from build123d import *

# Parameters (mm, degrees)
SKETCH1_W           = 120.65
SKETCH1_H           = 82.55
BOSS_EXTRUDE1_DEPTH = 12.7
FILLET1_R           = 16.002
SKETCH2_R           = 5.588
SKETCH2_R_2         = 3.231202494
SKETCH2_R_3         = 6.35
CUT_EXTRUDE1_DEPTH  = 12.7
BOSS_EXTRUDE2_START = 6.35
SKETCH2_5_W         = 25.4
SKETCH2_5_H         = 25.4
SKETCH2_5_R         = 6.35
BOSS_EXTRUDE2_DEPTH = 6.35
BOSS_EXTRUDE3_DEPTH = 25.4
BOSS_EXTRUDE4_DEPTH = 17.526
BOSS_EXTRUDE5_DEPTH = 12.7
FILLET2_R           = 3.175
FILLET3_R           = 3.175
FILLET4_R           = 3.175
SKETCH5_R           = 8.001
CUT_EXTRUDE2_DEPTH  = 4.572
SKETCH6_R           = 4.826
CUT_EXTRUDE3_DEPTH  = 25.654
SKETCH7_W           = 44.45
SKETCH7_H           = 12.7
CUT_EXTRUDE4_DEPTH  = 12.7
FILLET5_R           = 3.175
FILLET6_R           = 3.175
SKETCH8_R           = 3.175
CUT_EXTRUDE5_DEPTH  = 12.7


with BuildPart() as part:
    # Sketch1 → Boss-Extrude1 (new body)
    with BuildSketch(Plane(origin=(0, 0, 0), x_dir=(1, 0, 0), z_dir=(0, 1, 0))):
        Rectangle(SKETCH1_W, SKETCH1_H)
    extrude(amount=BOSS_EXTRUDE1_DEPTH)

    # Fillet1
    fillet1_edges = [part.edges().sort_by_distance(p)[0] for p in [
        (-60.325, 6.35, 41.275),
    ]]
    fillet(fillet1_edges, radius=FILLET1_R)

    # Sketch2 → Cut-Extrude1 (cut)
    with BuildSketch(Plane(origin=(0, 12.7, 0), x_dir=(1, 0, 0), z_dir=(0, 1, 0))):
        with Locations(Location((36.449, -9.525, 0), (0, 0, 270))):
            Circle(SKETCH2_R)
        with Locations(Location((36.449, -28.575, 0), (0, 0, 270))):
            Circle(SKETCH2_R)
        with Locations(Location((-9.525, 17.653, 0), (0, 0, 270))):
            Circle(SKETCH2_R_2)
        with Locations(Location((-44.323, -25.273, 0), (0, 0, 270))):
            Circle(SKETCH2_R)
        with Locations(Location((-3.175, -28.575, 0), (0, 0, 270))):
            Circle(SKETCH2_R_3)
        with BuildLine():
            Line((-47.625, 41.275), (-60.325, 41.275))
            Line((-60.325, 41.275), (-60.325, 28.575))
            ThreePointArc((-60.325, 28.575), (-51.344743879, 32.294743879), (-47.625, 41.275))
        make_face()
        with BuildLine():
            Line((-60.325, 3.175), (-31.877, 3.175))
            ThreePointArc((-31.877, 3.175), (-25.527, -3.175), (-31.877, -9.525))
            Line((-31.877, -9.525), (-60.325, -9.525))
            Line((-60.325, -9.525), (-60.325, 3.175))
        make_face()
    extrude(amount=-CUT_EXTRUDE1_DEPTH, mode=Mode.SUBTRACT)

    # Sketch2<5> → Boss-Extrude2 (add)
    with BuildSketch(Plane(origin=(0, 12.7, 0), x_dir=(1, 0, 0), z_dir=(0, 1, 0)).offset(BOSS_EXTRUDE2_START)):
        with Locations((-3.175, -28.575)):
            Rectangle(SKETCH2_5_W, SKETCH2_5_H)
        with Locations(Location((-3.175, -28.575, 0), (0, 0, 270))):
            Circle(SKETCH2_5_R, mode=Mode.SUBTRACT)
    extrude(amount=-BOSS_EXTRUDE2_DEPTH)

    # Sketch2<6> → Boss-Extrude3 (add)
    with BuildSketch(Plane(origin=(0, 12.7, 0), x_dir=(1, 0, 0), z_dir=(0, 1, 0))):
        Polygon((60.325, -41.275), (60.325, 41.275), (9.525, 41.275), (9.525, 28.575), (47.625, 28.575), (47.625, -41.275), align=None)
    extrude(amount=BOSS_EXTRUDE3_DEPTH)

    # Sketch2<10> → Boss-Extrude4 (add)
    with BuildSketch(Plane(origin=(0, 12.7, 0), x_dir=(1, 0, 0), z_dir=(0, 1, 0))):
        with BuildLine():
            Line((11.049, 28.575), (11.049, 14.351))
            ThreePointArc((11.049, 14.351), (23.749, 1.651), (36.449, 14.351))
            Line((36.449, 14.351), (36.449, 28.575))
            Line((36.449, 28.575), (11.049, 28.575))
        make_face()
    extrude(amount=BOSS_EXTRUDE4_DEPTH)

    # Sketch4 → Boss-Extrude5 (add)
    with BuildSketch(Plane(origin=(0, 0, -41.275), x_dir=(-1, 0, 0), z_dir=(0, 0, -1))):
        Polygon((-9.525, 38.1), (-9.525, 12.7), (34.469090512, 12.7), align=None)
    extrude(amount=-BOSS_EXTRUDE5_DEPTH)

    # Fillet2
    fillet2_edges = [part.edges().sort_by_distance(p)[0] for p in [
        (42.037, 12.7, -28.575),
        (36.449, 21.463, -28.575),
        (11.049, 12.7, -21.463),
        (11.049, 21.463, -28.575),
        (23.749, 12.7, -1.651),
        (36.449, 12.7, -21.463),
        (23.749, 30.226, -28.575),
        (-11.710045256, 12.7, -28.575),
        (47.625, 12.7, 6.35),
        (47.625, 25.4, -28.575),
    ]]
    fillet(fillet2_edges, radius=FILLET2_R)

    # Fillet3
    fillet3_edges = [part.edges().sort_by_distance(p)[0] for p in [
        (9.525, 15.875, 15.875),
        (-15.875, 15.875, 15.875),
        (-15.875, 15.875, 41.275),
        (9.525, 15.875, 41.275),
    ]]
    fillet(fillet3_edges, radius=FILLET3_R)

    # Fillet4
    # the kernel refuses this fillet: 3.175 mm, written as the material it adds along each edge
    with BuildSketch(Plane(origin=(9.525, 12.7, 19.05), x_dir=(0, 1, 0), z_dir=(0, 0, 1)), Plane(origin=(-12.7, 12.7, 15.875), x_dir=(0, 1, 0), z_dir=(1, 0, 0)), Plane(origin=(-15.875, 12.7, 38.1), x_dir=(0, 1, 0), z_dir=(0, 0, -1))) as fillet4_piece_1:
        with BuildLine():
            CenterArc((FILLET4_R, -FILLET4_R), FILLET4_R, 90, 90)
            Line((0, -FILLET4_R), (0, 0))
            Line((0, 0), (FILLET4_R, 0))
        make_face()
    extrude(amount=19.05)
    with BuildSketch(Plane(origin=(6.35, 12.7, 38.1), x_dir=(-0.5976672776328281, 0, -0.8017442392976478), z_dir=(0.8017442392976478, 0, -0.5976672776328281))) as fillet4_piece_2_section:
        with BuildLine():
            CenterArc((3.175 + FILLET4_R, FILLET4_R), FILLET4_R, 180, 90)
            Line((3.175 + FILLET4_R, 0), (3.175, 0))
            Line((3.175, 0), (3.175, FILLET4_R))
        make_face()
    fillet4_piece_2 = revolve(axis=Axis((6.35, 12.7, 38.1), (0, 1, 0)), revolution_arc=233.296989237, mode=Mode.PRIVATE)
    fillet4_piece_2 = split(fillet4_piece_2, bisect_by=Plane(origin=(8.731056041, 13.689420087, 41.275), z_dir=(0, 0, -1)), keep=Keep.TOP, mode=Mode.PRIVATE)
    add(fillet4_piece_2)
    with BuildSketch(Plane(origin=(6.35, 12.7, 19.05), x_dir=(0, 0, -1), z_dir=(-1, 0, 0))) as fillet4_piece_3:
        with BuildLine():
            CenterArc((3.175 + FILLET4_R, -FILLET4_R), FILLET4_R, 90, 90)
            Line((3.175 + FILLET4_R, 0), (3.175, 0))
            Line((3.175, 0), (3.175, -FILLET4_R))
        make_face()
    revolve(axis=Axis((6.35, 12.7, 19.05), (0, -1, 0)), revolution_arc=90)
    with BuildSketch(Plane(origin=(-12.7, 12.7, 19.05), x_dir=(-1, 0, 0), z_dir=(0, 0, 1))) as fillet4_piece_4:
        with BuildLine():
            CenterArc((3.175 + FILLET4_R, -FILLET4_R), FILLET4_R, 90, 90)
            Line((3.175 + FILLET4_R, 0), (3.175, 0))
            Line((3.175, 0), (3.175, -FILLET4_R))
        make_face()
    revolve(axis=Axis((-12.7, 12.7, 19.05), (0, -1, 0)), revolution_arc=90)
    with BuildSketch(Plane(origin=(-12.7, 12.7, 38.1), x_dir=(0.5976672776328279, 0, -0.8017442392976479), z_dir=(-0.8017442392976479, 0, -0.5976672776328279))) as fillet4_piece_5_section:
        with BuildLine():
            CenterArc((3.175 + FILLET4_R, -FILLET4_R), FILLET4_R, 90, 90)
            Line((3.175, -FILLET4_R), (3.175, 0))
            Line((3.175, 0), (3.175 + FILLET4_R, 0))
        make_face()
    fillet4_piece_5 = revolve(axis=Axis((-12.7, 12.7, 38.1), (0, -1, 0)), revolution_arc=233.296989237, mode=Mode.PRIVATE)
    fillet4_piece_5 = split(fillet4_piece_5, bisect_by=Plane(origin=(-15.081056252, 13.689419911, 41.275), z_dir=(0, 0, -1)), keep=Keep.TOP, mode=Mode.PRIVATE)
    add(fillet4_piece_5)

    # Sketch5 → Cut-Extrude2 (cut)
    with BuildSketch(Plane(origin=(0, 30.226, 0), x_dir=(1, 0, 0), z_dir=(0, 1, 0))):
        with Locations(Location((23.749, 14.351, 0), (0, 0, 270))):
            Circle(SKETCH5_R)
    extrude(amount=-CUT_EXTRUDE2_DEPTH, mode=Mode.SUBTRACT)

    # Sketch6 → Cut-Extrude3 (cut)
    with BuildSketch(Plane(origin=(0, 25.654, 0), x_dir=(1, 0, 0), z_dir=(0, 1, 0))):
        with Locations(Location((23.749, 14.351, 0), (0, 0, 270))):
            Circle(SKETCH6_R)
    extrude(amount=-CUT_EXTRUDE3_DEPTH, mode=Mode.SUBTRACT)

    # Sketch7 → Cut-Extrude4 (cut)
    with BuildSketch(Plane(origin=(60.325, 0, 0), x_dir=(0, 0, -1), z_dir=(1, 0, 0))):
        with Locations((0, 31.75)):
            Rectangle(SKETCH7_W, SKETCH7_H)
    extrude(amount=-CUT_EXTRUDE4_DEPTH, mode=Mode.SUBTRACT)

    # Fillet5
    fillet5_edges = [part.edges().sort_by_distance(p)[0] for p in [
        (53.975, 38.1, -22.225),
    ]]
    fillet(fillet5_edges, radius=FILLET5_R)

    # Fillet6
    fillet6_edges = [part.edges().sort_by_distance(p)[0] for p in [
        (53.975, 38.1, 22.225),
        (53.975, 38.1, 41.275),
    ]]
    fillet(fillet6_edges, radius=FILLET6_R)

    # Sketch8 → Cut-Extrude5 (cut)
    with BuildSketch(Plane(origin=(60.325, 0, 0), x_dir=(0, 0, -1), z_dir=(1, 0, 0))):
        with Locations((-31.75, 25.4)):
            Circle(SKETCH8_R)
    extrude(amount=-CUT_EXTRUDE5_DEPTH, mode=Mode.SUBTRACT)


solid = part.part
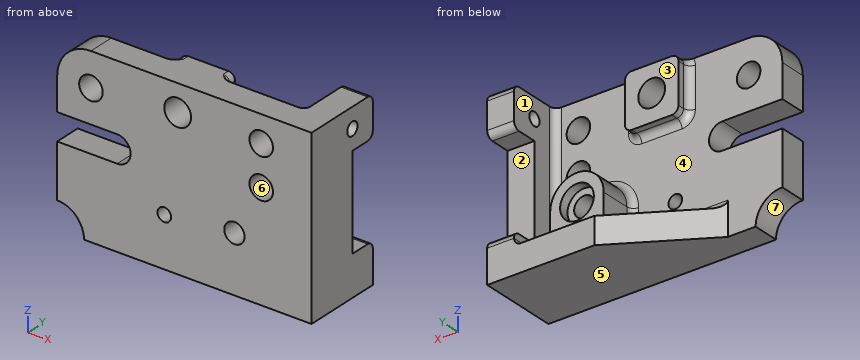
Here's how the part is built. I have some questions about the finished solid (model axes, mm). Face numbers are marked on the shaded views. A direction names the side the tool comes from. Coordinates: 2 decimals unless noted, no trailing zeros. Order: outer loops, then holes, each group sorted by start corner. A loop starts at its lowest first (then second) coordinate and runs counter-clockwise, first axis right, second up. Notation, with made-up numbers: (-7.75, 5) - (49.25, 5) arc R18 ccw to (49.25, 35) - close; hole circle Ø4 at (-2.5, 47). An arc over 180 degrees is marked (long way). Use CSV: the item, a comma, the result in double quotes. Start each with the question number.
1. For the marked faces 1, 2, 3 and 4, which set-ups out of +Z, -Z, +X, -X, +Y, -Y let a thin tool reach every point of the face, with its end or its side?
2. Suppose I cut it at C-C on z = -17. List the corners of the cut face in (x, y) for me (3 decimals).
3. Suppose I cut it at A-A on z = 6.5. List the corners of the cut face in (x, y) for me (3 decimals).
4. If we mould it in two halves opening along X, with no side actions, what happens to the marked faces 5, 6 and 7? For each: +X half, -X half, draft (parallel to the pull), parting line (faces both ways), or undercut.
5. Please list where these lines run through material, in increasing order: line 1 (Z direction, x = 23.5, y = 2) (3 decimals); line 2 (X direction, y = 18, z = 38) (3 decimals); line 3 (X direction, y = 5.5, z = -16) (3 decimals). Write a range as from..to.
6. I'm going to push flat-ended pins straight in: pin 1 (20.5 mm diameter, centred on x = -2, z = 26, fed in from +Y); pin 2 (17.5 mm diameter, centred on x = 23, z = -12, fed in from +Y); pin 3 (2.5 mm diameter, centred on y = 17, z = 31.5, fed in from -X); pin 4 (10 mm diameter, centred on x = -3.175, z = 28.575, fed in from +Y). Where does each tip first touch, or does it pass through?
7. Suppose I cut it at B-B on x = -43. List the corners of the cut face in (y, z) for me (3 decimals), then the cut area to 3 significant figures.
Output:
1,face 1,"+Z, +Y"
1,face 2,"+X, +Y"
1,face 3,"+Z, -X, +Y"
1,face 4,"+Y"
2,outline,"(-60.325, 0) - (-12.69, 0) - (-12.69, 12.7) - (-60.325, 12.7) - close; (-6.36, 0) - (19.715, 0) - (19.715, 25.654) - (16.199, 25.654) - (16.199, 30.226) - (11.049, 30.226) - (11.049, 15.875) arc R3.175 cw to (7.874, 12.7) - (-6.36, 12.7) - close; (27.783, 0) - (60.325, 0) - (60.325, 25.4) - (47.625, 25.4) - (47.625, 15.875) arc R3.175 cw to (44.45, 12.7) - (39.624, 12.7) arc R3.175 cw to (36.449, 15.875) - (36.449, 30.226) - (31.299, 30.226) - (31.299, 25.654) - (27.783, 25.654) - close"
3,outline,"(-26.467, 0) - (31.751, 0) - (31.751, 12.7) - (-26.467, 12.7) - close; (41.147, 0) - (60.325, 0) - (60.325, 25.4) - (47.625, 25.4) - (47.625, 15.875) arc R3.175 cw to (44.45, 12.7) - (41.147, 12.7) - close"
4,face 5,"draft"
4,face 6,"undercut"
4,face 7,"-X half"
5,line 1,"z = -41.275..-19.171, -9.531..41.275"
5,line 2,"x = -15.875..9.525, 47.625..60.325"
5,line 3,"x = -60.325..-12.301, -6.749..19.213, 28.285..60.325"
6,pin 1,"stops at y = 19.05"
6,pin 2,"stops at y = 30.23"
6,pin 3,"stops at x = -15.88"
6,pin 4,"passes through"
7,outline,"(0, -41.275) - (12.7, -41.275) - (12.7, -3.175) - (0, -3.175) - close; (0, 9.525) - (12.7, 9.525) - (12.7, 19.844) - (0, 19.844) - close; (0, 30.702) - (12.7, 30.702) - (12.7, 41.275) - (0, 41.275) - close"
7,area,"749 mm2"
